Here's how the part is built. I have some questions about the finished solid (model axes, mm). A direction names the side the tool comes from. Round coordinates to 2 decimals unless told otherwise and drop trailing zeros. Write each loop counter-clockwise with the first axis right and the second up, starting at its lowest first coordinate (ties: lowest second). Pieces come first, ordered by that corner, then holes. Notation, with made-up numbers: (7.5, 30.25) -> (54.5, 30.25) arc R15 ccw to (54.5, 51.25) -> close; hole circle Ø7 at (8.25, 68). An arc over 180 degrees is marked (long way). Answer as CSV lines item,"result".
```python
from build123d import *

# Parameters (mm, degrees)
SKETCH1_R               = 20.828
SKETCH1_R_2             = 2.1
BOSS_EXTRUDE1_DEPTH     = 7.9248
CUT_EXTRUDE1_DEPTH      = 6.4008
SKETCH3_R               = 2.52095
SKETCH3_R_2             = 0.99695
BOSS_EXTRUDE2_DEPTH     = 6.4008
SKETCH4_R               = 0.99695
CUT_EXTRUDE2_DEPTH      = 69.690466883
SKETCH5_R               = 20.828
SKETCH5_R_2             = 0.99695
BOSS_EXTRUDE3_DEPTH     = 6.4008
BOSS_EXTRUDE4_DEPTH     = 7.9248
CUT_EXTRUDE3_REACH      = 114.995
CUT_EXTRUDE3_END_RADIUS = 22.225
SKETCH7_R               = 2.2606
CUT_EXTRUDE4_DEPTH      = 5
FILLET1_R               = 12.7
CUT_EXTRUDE5_DEPTH      = 60.706


with BuildPart() as part:
    # Sketch1 → Boss-Extrude1 (new body)
    with BuildSketch(Plane(origin=(0, 0, 0), x_dir=(1, 0, 0), z_dir=(0, 1, 0))):
        with BuildLine():
            Line((-19.05, -25.4), (57.15, -25.4))
            ThreePointArc((57.15, -25.4), (61.640128061, -23.540128061), (63.5, -19.05))
            Line((63.5, -19.05), (63.5, 19.05))
            ThreePointArc((63.5, 19.05), (61.640128061, 23.540128061), (57.15, 25.4))
            Line((57.15, 25.4), (-19.05, 25.4))
            ThreePointArc((-19.05, 25.4), (-23.540128061, 23.540128061), (-25.4, 19.05))
            Line((-25.4, 19.05), (-25.4, -19.05))
            ThreePointArc((-25.4, -19.05), (-23.540128061, -23.540128061), (-19.05, -25.4))
        make_face()
        with Locations(Location((38.1, 0, 0), (0, 0, 270))):
            Circle(SKETCH1_R, mode=Mode.SUBTRACT)
        with Locations(Location((-19.05, 19.05, 0), (0, 0, 270))):
            Circle(SKETCH1_R_2, mode=Mode.SUBTRACT)
        with Locations(Location((-19.05, -19.05, 0), (0, 0, 270))):
            Circle(SKETCH1_R_2, mode=Mode.SUBTRACT)
        with Locations(Location((57.15, -19.05, 0), (0, 0, 270))):
            Circle(SKETCH1_R_2, mode=Mode.SUBTRACT)
        with Locations(Location((57.15, 19.05, 0), (0, 0, 270))):
            Circle(SKETCH1_R_2, mode=Mode.SUBTRACT)
    extrude(amount=BOSS_EXTRUDE1_DEPTH)

    # Sketch2 → Cut-Extrude1 (cut)
    with BuildSketch(Plane(origin=(0, 7.9248, 0), x_dir=(1, 0, 0), z_dir=(0, 1, 0))):
        with BuildLine():
            Line((0, 22.225), (38.1, 22.225))
            ThreePointArc((38.1, 22.225), (60.325, 0), (38.1, -22.225))
            Line((38.1, -22.225), (0, -22.225))
            ThreePointArc((0, -22.225), (-22.225, 0), (0, 22.225))
        make_face()
    extrude(amount=-CUT_EXTRUDE1_DEPTH, mode=Mode.SUBTRACT)

    # Sketch3 → Boss-Extrude2 (add)
    # profile 1 of 4: a face of its own
    with BuildSketch(Plane(origin=(0, 1.524, 0), x_dir=(1, 0, 0), z_dir=(0, 1, 0))):
        with Locations(Location((-5.08, 8.636, 0), (0, 0, 90))):
            Circle(SKETCH3_R)
        with Locations(Location((-5.08, 8.636, 0), (0, 0, 90))):
            Circle(SKETCH3_R_2, mode=Mode.SUBTRACT)
    # profile 2 of 4: a face of its own
    with BuildSketch(Plane(origin=(0, 1.524, 0), x_dir=(1, 0, 0), z_dir=(0, 1, 0))):
        with Locations(Location((5.08, 8.636, 0), (0, 0, 90))):
            Circle(SKETCH3_R)
        with Locations(Location((5.08, 8.636, 0), (0, 0, 90))):
            Circle(SKETCH3_R_2, mode=Mode.SUBTRACT)
    # profile 3 of 4: a face of its own
    with BuildSketch(Plane(origin=(0, 1.524, 0), x_dir=(1, 0, 0), z_dir=(0, 1, 0))):
        with Locations(Location((5.08, -8.636, 0), (0, 0, 90))):
            Circle(SKETCH3_R)
        with Locations(Location((5.08, -8.636, 0), (0, 0, 90))):
            Circle(SKETCH3_R_2, mode=Mode.SUBTRACT)
    # profile 4 of 4: a face of its own
    with BuildSketch(Plane(origin=(0, 1.524, 0), x_dir=(1, 0, 0), z_dir=(0, 1, 0))):
        with Locations(Location((-5.08, -8.636, 0), (0, 0, 90))):
            Circle(SKETCH3_R)
        with Locations(Location((-5.08, -8.636, 0), (0, 0, 90))):
            Circle(SKETCH3_R_2, mode=Mode.SUBTRACT)
    extrude(amount=BOSS_EXTRUDE2_DEPTH)

    # Sketch4 → Cut-Extrude2 (cut, through all)
    with BuildSketch(Plane(origin=(0, 1.524, 0), x_dir=(1, 0, 0), z_dir=(0, 1, 0))):
        with Locations(Location((5.08, -8.636, 0), (0, 0, 90))):
            Circle(SKETCH4_R)
        with Locations(Location((-5.08, -8.636, 0), (0, 0, 90))):
            Circle(SKETCH4_R)
        with Locations(Location((5.08, 8.636, 0), (0, 0, 90))):
            Circle(SKETCH4_R)
        with Locations(Location((-5.08, 8.636, 0), (0, 0, 90))):
            Circle(SKETCH4_R)
    extrude(amount=-CUT_EXTRUDE2_DEPTH, mode=Mode.SUBTRACT)

    # Sketch5 → Boss-Extrude3 (add)
    with BuildSketch(Plane(origin=(0, 1.524, 0), x_dir=(1, 0, 0), z_dir=(0, 1, 0))):
        with BuildLine():
            Line((0, 22.225), (0, -22.225))
            Line((0, -22.225), (38.1, -22.225))
            ThreePointArc((38.1, -22.225), (60.325, 0), (38.1, 22.225))
            Line((38.1, 22.225), (0, 22.225))
        make_face()
        with Locations(Location((38.1, 0, 0), (0, 0, 90))):
            Circle(SKETCH5_R, mode=Mode.SUBTRACT)
        with Locations(Location((5.08, -8.636, 0), (0, 0, 90))):
            Circle(SKETCH5_R_2, mode=Mode.SUBTRACT)
        with Locations(Location((5.08, 8.636, 0), (0, 0, 90))):
            Circle(SKETCH5_R_2, mode=Mode.SUBTRACT)
    extrude(amount=BOSS_EXTRUDE3_DEPTH)

    # Sketch6 → Boss-Extrude4 (add)
    with BuildSketch(Plane.XZ):
        with BuildLine():
            Line((42.8625, 66.217346987), (62.939460474, 21.658571912))
            ThreePointArc((62.939460474, 21.658571912), (60.596597479, 24.383241587), (57.15, 25.4))
            Line((57.15, 25.4), (14.945483896, 25.4))
            Line((14.945483896, 25.4), (33.3375, 66.217346987))
            ThreePointArc((33.3375, 66.217346987), (35.264775446, 68.45870253), (38.1, 69.295103774))
            ThreePointArc((38.1, 69.295103774), (40.935224554, 68.45870253), (42.8625, 66.217346987))
        make_face()
        with BuildLine():
            Line((57.15, -25.4), (14.945483896, -25.4))
            Line((14.945483896, -25.4), (33.3375, -66.217346987))
            ThreePointArc((33.3375, -66.217346987), (35.264775446, -68.45870253), (38.1, -69.295103774))
            ThreePointArc((38.1, -69.295103774), (40.935224554, -68.45870253), (42.8625, -66.217346987))
            Line((42.8625, -66.217346987), (62.939460474, -21.658571912))
            ThreePointArc((62.939460474, -21.658571912), (60.596597479, -24.383241587), (57.15, -25.4))
        make_face()
    extrude(amount=-BOSS_EXTRUDE4_DEPTH)

    # Cut-Extrude3: up to this cylinder (the profile starts outside it)
    cut_extrude3_end = Plane(origin=(0, 7.9248, 0), z_dir=(0, 1, 0)) * Cylinder(CUT_EXTRUDE3_END_RADIUS, 275.44, mode=Mode.PRIVATE)
    # Sketch7 → Cut-Extrude3 (cut, up to the surface)
    with BuildSketch(Plane.ZY.offset(25.4), mode=Mode.PRIVATE) as cut_extrude3_sk1:
        with Locations((0, 7.9248)):
            Circle(SKETCH7_R)
    cut_extrude3_tool1 = extrude(cut_extrude3_sk1.sketch, amount=-CUT_EXTRUDE3_REACH, mode=Mode.PRIVATE) - cut_extrude3_end
    add(cut_extrude3_tool1.solids().sort_by_distance((-25.4, 7.9248, 0))[0], mode=Mode.SUBTRACT)

    # Sketch8 → Cut-Extrude4 (cut)
    with BuildSketch(Plane.XZ):
        Polygon((-17.000406544, 22.6), (-21.099593456, 22.6), (-23.149186911, 19.05), (-21.099593456, 15.5), (-17.000406544, 15.5), (-14.950813089, 19.05), align=None)
        Polygon((-17.000406544, -15.5), (-21.099593456, -15.5), (-23.149186911, -19.05), (-21.099593456, -22.6), (-17.000406544, -22.6), (-14.950813089, -19.05), align=None)
        Polygon((59.199593456, -15.5), (55.100406544, -15.5), (53.050813089, -19.05), (55.100406544, -22.6), (59.199593456, -22.6), (61.249186911, -19.05), align=None)
        Polygon((59.199593456, 22.6), (55.100406544, 22.6), (53.050813089, 19.05), (55.100406544, 15.5), (59.199593456, 15.5), (61.249186911, 19.05), align=None)
    extrude(amount=-CUT_EXTRUDE4_DEPTH, mode=Mode.SUBTRACT)

    # Fillet1
    fillet1_edges = [part.edges().sort_by_distance(p)[0] for p in [
        (14.945483896, 3.9624, 25.4),
        (14.945483896, 3.9624, -25.4),
    ]]
    fillet(fillet1_edges, radius=FILLET1_R)

    # Sketch9 → Cut-Extrude5 (cut)
    with BuildSketch(Plane(origin=(0, 7.9248, 0), x_dir=(1, 0, 0), z_dir=(0, 1, 0))):
        with BuildLine():
            Line((34.9123, -63.5), (34.9123, -48.26))
            ThreePointArc((34.9123, -48.26), (38.1, -45.0723), (41.2877, -48.26))
            Line((41.2877, -48.26), (41.2877, -63.5))
            ThreePointArc((41.2877, -63.5), (38.1, -66.6877), (34.9123, -63.5))
        make_face()
        with BuildLine():
            Line((41.2877, 63.5), (41.2877, 48.26))
            ThreePointArc((41.2877, 48.26), (38.1, 45.0723), (34.9123, 48.26))
            Line((34.9123, 48.26), (34.9123, 63.5))
            ThreePointArc((34.9123, 63.5), (38.1, 66.6877), (41.2877, 63.5))
        make_face()
    extrude(amount=-CUT_EXTRUDE5_DEPTH, mode=Mode.SUBTRACT)


solid = part.part
```
1. Suppose I cut it at A-A on y = 3.5. Count the separate pieces of the cut face and the enclosed holes in it, and give its area (3 significant figures).
Numbers:
separate pieces,"3"
enclosed holes,"12"
area,"4,290 mm^2"
2. Suppose I cut it at D-D on x = 57.15. Please give me the cut outline in (y, z), and give its area (3 significant figures).
Numbers:
outline,"(0, -34.51) -> (7.92, -34.51) -> (7.92, -21.15) -> (5, -21.15) -> (5, -22.6) -> (0, -22.6) -> close; (0, -15.5) -> (5, -15.5) -> (5, -16.95) -> (7.92, -16.95) -> (7.92, -8.42) -> (0, -8.42) -> close; (0, 8.42) -> (7.92, 8.42) -> (7.92, 16.95) -> (5, 16.95) -> (5, 15.5) -> (0, 15.5) -> close; (0, 22.6) -> (5, 22.6) -> (5, 21.15) -> (7.92, 21.15) -> (7.92, 34.51) -> (0, 34.51) -> close"
area,"318 mm^2"
3. Suppose I cut it at B-B on x = 26. Please give me the cut outline in (y, z), and give its area (3 significant figures).
Numbers:
outline,"(0, -49.93) -> (7.92, -49.93) -> (7.92, -16.95) -> (0, -16.95) -> close; (0, 16.95) -> (7.92, 16.95) -> (7.92, 49.93) -> (0, 49.93) -> close"
area,"523 mm^2"
4. If I drill on line 1 (Z direction, x = -5, y = 4); line 2 (Z direction, x = -5.08, y = 0.7); line 3 (Z direction, x = 54, y = 4.75), over which ranges is the centre line in solid material (lowest first)?
Numbers:
line 1,"z = -25.4 to -21.66, -11.16 to -9.63, -7.64 to -6.12, 6.12 to 7.64, 9.63 to 11.16, 21.66 to 25.4"
line 2,"z = -25.4 to -9.63, -7.64 to 7.64, 9.63 to 25.4"
line 3,"z = -41.5 to -20.69, -17.41 to -13.45, 13.45 to 17.41, 20.69 to 41.5"
5. For pin 1 Ø4.5 at (x, y) = (-19, 3) entering from -Z; pin 2 Ø6 at (x, z) = (39.5, -54.5) entering from -Y; pin 3 Ø4.5 at (x, y) = (57.5, 2.5) entering from +Z; pin 4 Ø1 at (x, y) = (0, 5.5) entering from +Z, each with a flat end and sliding along its axis, tell me the tip position at first contact or that it passes through.
Numbers:
pin 1,"stops at z = -25.4"
pin 2,"stops at y = 0"
pin 3,"stops at z = 38.72"
pin 4,"stops at z = 25.4"
6. If we mould it in two halves opening along X, with no side actions, what happens to faces 5 (the face through (-6, 4, 25.4)), 6 (the face through (54.09, 2.46, 20.85)), 7 (the face through (25.722, 3.907, -49.317)), 8 (the face through (-19, 2, 22.6))? For each: released by +X, released by -X, zero draft, split by the parting line, or undercut.
Numbers:
face 5,"zero draft"
face 6,"undercut"
face 7,"released by -X"
face 8,"undercut"
7. Suppose I cut it at C-C on z = 54. Please give me the cut outline in (x, y).
Numbers:
outline,"(27.83, 0) -> (34.91, 0) -> (34.91, 7.92) -> (27.83, 7.92) -> close; (41.29, 0) -> (48.37, 0) -> (48.37, 7.92) -> (41.29, 7.92) -> close"
8. On a 3-axis mill with a long thin cutter (end or side, diameter ignored), from which of +Z, -Z, +X, -X, +Y, -Y can I reach the whole of each face in a straight line? I mean faces 1 (the face through (54.09, 2.46, -17.25)), 2 (the face through (41.288, 4, 56)), 3 (the face through (-6, 4, -25.4)), 4 (the face through (-23.778, 5.665, -0.05)). Say none if no direction works.
Numbers:
face 1,"-Y"
face 2,"+Y, -Y"
face 3,"-Z, -X, +Y, -Y"
face 4,"-X, +Y"
